from build123d import *

# Parameters (mm, degrees)
SKETCH1_W           = 75
SKETCH1_H           = 20
BOSS_EXTRUDE1_DEPTH = 1
CUT_EXTRUDE1_DEPTH  = 39.823317736
FILLET1_R           = 1
FILLET2_R           = 1
SKETCH3_W           = 15
SKETCH3_H           = 3
CUT_EXTRUDE2_DEPTH  = 1.25


with BuildPart() as part:
    # Sketch1 → Boss-Extrude1 (new body)
    with BuildSketch(Plane.XY):
        Rectangle(SKETCH1_W, SKETCH1_H)
    extrude(amount=BOSS_EXTRUDE1_DEPTH)

    # Sketch2 → Cut-Extrude1 (cut, through all)
    with BuildSketch(Plane.XY.offset(1)):
        with BuildLine():
            Line((-37.5, 6), (-24.5, 6))
            Line((-24.5, 6), (-24.5, -6))
            Line((-24.5, -6), (-37.5, -6))
            ThreePointArc((-37.5, -6), (-43.5, 0), (-37.5, 6))
        make_face()
    cut_extrude1 = extrude(amount=-CUT_EXTRUDE1_DEPTH, mode=Mode.SUBTRACT)

    # Fillet1
    fillet1_edges = [part.edges().sort_by_distance(p)[0] for p in [
        (-37.5, -6, 0.5),
        (-37.5, 6, 0.5),
        (-24.5, 6, 0.5),
        (-24.5, -6, 0.5),
        (-37.5, 10, 0.5),
        (-37.5, -10, 0.5),
    ]]
    fillet(fillet1_edges, radius=FILLET1_R)

    # Mirror1: Cut-Extrude1 across plane
    add(cut_extrude1.mirror(Plane(origin=(0, 0, 0), x_dir=(0, 0, 1), z_dir=(1, 0, 0))), mode=Mode.SUBTRACT)

    # Fillet2
    fillet2_edges = [part.edges().sort_by_distance(p)[0] for p in [
        (37.5, 6, 0.5),
        (37.5, -6, 0.5),
        (24.5, -6, 0.5),
        (24.5, 6, 0.5),
        (37.5, 10, 0.5),
        (37.5, -10, 0.5),
    ]]
    fillet(fillet2_edges, radius=FILLET2_R)

    # Sketch3 → Cut-Extrude2 (cut)
    with BuildSketch(Plane.XY.offset(1)):
        Rectangle(SKETCH3_W, SKETCH3_H)
    extrude(amount=-CUT_EXTRUDE2_DEPTH, mode=Mode.SUBTRACT)


solid = part.part
Could you check a few things on this model? Use its own coordinates, in mm. Give positions to 0.01 mm unless a question says otherwise; leave off trailing zeros. Order: outer loops, then holes, each group sorted by start corner. A loop starts at its lowest first (then second) coordinate and runs counter-clockwise, first axis right, second up.
1. Suppose I cut it at D-D (y = 3.5). List the corners of the cut face in (x, z) for me, plus the area to 3 significant figures.
2. Suppose I cut it at A-A (x = 32). List the corners of the cut face in (y, z) for me, plus the area to 3 significant figures.
3. Will these pins go through, and if not, where does the flat tip stop? P1, Ø6, axis at x = -21, y = 0, coming from the -Z side; P2, Ø0.5, axis at y = -1.5, z = 0.5, coming from the -X side.
4. I need wall thicknesses on L1, parallel to Y at x = 3, z = 0.7; L2, parallel to Y at x = 27.5, z = 0.5; L3, parallel to X at y = 3.5, z = 0.7. Which ranges of each line are inside material? Lowest first, please.
5. Suppose I cut it at B-B (z = 0.3). List the corners of the cut face in (x, y) for me.
6. Suppose I cut it at C-C (y = 0.25). List the corners of the cut face in (x, z) for me, plus the area to 3 significant figures.
Solved:
1. outline: (-24.5, 0) - (24.5, 0) - (24.5, 1) - (-24.5, 1) - close
1. area: 49.0 mm2
2. outline: (-10, 0) - (-6, 0) - (-6, 1) - (-10, 1) - close; (6, 0) - (10, 0) - (10, 1) - (6, 1) - close
2. area: 8.00 mm2
3. P1: stops at z = 0
3. P2: stops at x = -24.5
4. L1: y = -10 to -1.5, 1.5 to 10
4. L2: y = -10 to -6, 6 to 10
4. L3: x = -24.5 to 24.5
5. outline: (-37.5, -9) arc R1 ccw to (-36.5, -10) - (36.5, -10) arc R1 ccw to (37.5, -9) - (37.5, -7) arc R1 ccw to (36.5, -6) - (25.5, -6) arc R1 cw to (24.5, -5) - (24.5, 5) arc R1 cw to (25.5, 6) - (36.5, 6) arc R1 ccw to (37.5, 7) - (37.5, 9) arc R1 ccw to (36.5, 10) - (-36.5, 10) arc R1 ccw to (-37.5, 9) - (-37.5, 7) arc R1 ccw to (-36.5, 6) - (-25.5, 6) arc R1 cw to (-24.5, 5) - (-24.5, -5) arc R1 cw to (-25.5, -6) - (-36.5, -6) arc R1 ccw to (-37.5, -7) - close; hole (-7.5, -1.5) - (7.5, -1.5) - (7.5, 1.5) - (-7.5, 1.5) - close
6. outline: (-24.5, 0) - (-7.5, 0) - (-7.5, 1) - (-24.5, 1) - close; (7.5, 0) - (24.5, 0) - (24.5, 1) - (7.5, 1) - close
6. area: 34.0 mm2
